Check sheet for the drawn part. Datum: minimum x, y, z corner. Units: mm. A direction names the side the tool comes from. Give positions to 0.01 mm unless a question says otherwise; leave off trailing zeros. Write each loop counter-clockwise with the first axis right and the second up, starting at its lowest first coordinate (ties: lowest second). Pieces come first, ordered by that corner, then holes. Notation, with made-up numbers: M 85,32 L 144,32 A13 ccw 144,40 Z; hole C 57.5,-33 d7. An arc over 180 degrees is marked long. Write item = value, one per line. Start each with the question number.
1) Sectioned sample at A-A, the plane x = 131.5. Record the cut outline in (y, z).
2) Sectioned sample at D-D, the plane z = 38. Record the cut outline in (x, y), then the cut area to 3 significant figures.
3) Scan lines: L1, parallel to X at y = 4.25, z = 5; L2, parallel to X at y = 7.5, z = 49; L3, parallel to Z at x = 139.5, y = 5. Record each from-to range of solid material in increasing order.
4) Draft check along X on the marked faces 1, 2 and 3. Enter one of: pulls with the +X half, pulls with the -X half, needs draft (parallel to the pull), parting line crosses it, or undercut.
5) Sectioned sample at B-B, the plane z = 30. Record the cut outline in (x, y), then the cut area to 3 significant figures.
6) Gauge pin test, flat ends, axial feed: pin 1 (3 mm diameter, centred on x = 33.5, z = 10.5, fed in from +Y); pin 2 (1 mm diameter, centred on x = 29.5, z = 28.5, fed in from +Y); pin 3 (2 mm diameter, centred on y = 13, z = 21, fed in from -X); pin 4 (8.5 mm diameter, centred on x = 9.5, z = 27, fed in from +Y). Record the tip position at first contact, or that the pin passes through.
7) Sectioned sample at C-C, the plane y = 16.75. Record the cut outline in (x, z).
8) Set-up check for the marked faces 4, 5 and 6: record each of +Z, -Z, +X, -X, +Y, -Y from which the full face is reachable in a straight line by a thin tool's end or side.
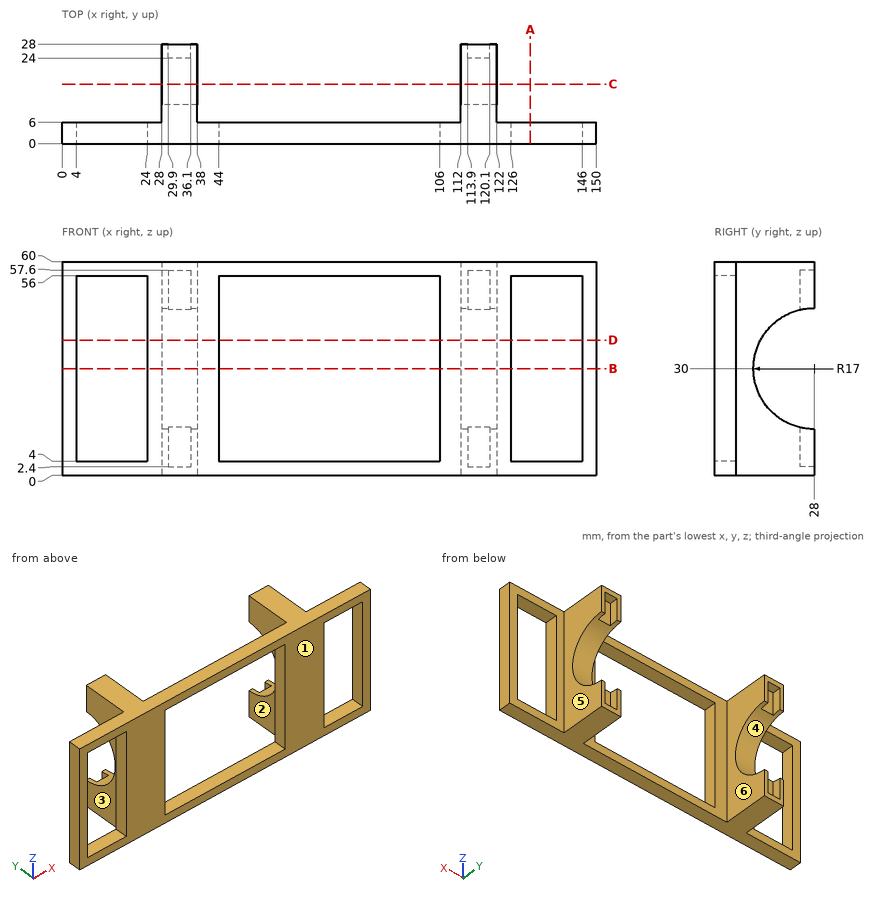
Data:
q1.outline = M 0,0 L 6,0 L 6,4 L 0,4 Z; M 0,56 L 6,56 L 6,60 L 0,60 Z
q2.outline = M 0,0 L 4,0 L 4,6 L 0,6 Z; M 24,0 L 44,0 L 44,6 L 38,6 L 38,13 L 28,13 L 28,6 L 24,6 Z; M 106,0 L 126,0 L 126,6 L 122,6 L 122,13 L 112,13 L 112,6 L 106,6 Z; M 146,0 L 150,0 L 150,6 L 146,6 Z
q2.area = 428 mm2
q3.L1 = 0 to 4, 24 to 44, 106 to 126, 146 to 150
q3.L2 = 28 to 38, 112 to 122
q3.L3 = 0 to 4, 56 to 60
q4.face_1 = needs draft
q4.face_2 = undercut
q4.face_3 = pulls with the -X half
q5.outline = M 0,0 L 4,0 L 4,6 L 0,6 Z; M 24,0 L 44,0 L 44,6 L 38,6 L 38,11 L 28,11 L 28,6 L 24,6 Z; M 106,0 L 126,0 L 126,6 L 122,6 L 122,11 L 112,11 L 112,6 L 106,6 Z; M 146,0 L 150,0 L 150,6 L 146,6 Z
q5.area = 388 mm2
q6.pin_1 = 24
q6.pin_2 = 11.12
q6.pin_3 = 28
q6.pin_4 = through
q7.outline = M 28,0 L 38,0 L 38,17.25 L 28,17.25 Z; M 28,42.75 L 38,42.75 L 38,60 L 28,60 Z; M 112,0 L 122,0 L 122,17.25 L 112,17.25 Z; M 112,42.75 L 122,42.75 L 122,60 L 112,60 Z
q8.face_4 = +X, -X, +Y
q8.face_5 = +Z, -Z, +X, +Y
q8.face_6 = +Z, -Z, +Y
